Could you check a few things on this model? Use its own coordinates, in mm. A direction names the side the tool comes from. Give positions to 0.01 mm unless a question says otherwise; leave off trailing zeros. Loops run counter-clockwise (first coordinate to the right, second up) from the corner with the lowest first, then second, coordinate; pieces in that order, holes last. Notation, with made-up numbers: (22, 57.5) -> (73, 57.5) arc R27 ccw to (73, 95.5) -> close; hole circle Ø2 at (58, 33.5). An arc over 180 degrees is marked (long way). Write item = value, one per line. Start each with the question number.
1) I want a section at D-D (z = -11). List the corners of the cut face in (x, y) for me (3 decimals).
2) I'm going to push flat-ended pins straight in: pin 1 Ø3 at (x, z) = (15.875, -6.35) entering from -Y; pin 2 Ø5 at (x, y) = (35.5, 31.5) entering from -Z. Where does each tip first touch, or does it pass through?
3) I want a section at B-B (y = 24.13). List the corners of the cut face in (x, z) for me (3 decimals).
4) I want a section at C-C (x = 6.35). List the corners of the cut face in (y, z) for me (3 decimals), and give its area (3 significant figures).
5) On a 3-axis mill with a long thin cutter (end or side, diameter ignored), from which of +Z, -Z, +X, -X, +Y, -Y can I reach the whole of each face in a straight line? I mean faces 1 (the face through (6, 6, -10.16)), 2 (the face through (38.1, 25, -19)), 3 (the face through (6.6, 45.07, -12.88)), 4 (the face through (14.015, 8.766, -5.937)). Say none if no direction works.
6) I need wall thicknesses on probe 1 along Y at (x, z) = (6.35, -16.75) (3 decimals); probe 2 along X at (y, z) = (47, -18.5); probe 3 along X at (y, z) = (6.5, -15). Which ranges of each line are inside material? Lowest first, please. Write a range as from..to.
7) If we mould it in two halves opening along X, with no side actions, what happens to faces 5 (the face through (35, 25, -12.7)), 6 (the face through (25.49, 29.32, -17.54)), 7 (the face through (50.8, 25, -13))? For each: +X half, -X half, draft (parallel to the pull), parting line (faces both ways), or undercut.
8) I want a section at A-A (z = -16.5). Count the separate pieces of the cut face and the enclosed holes in it, and give its area (3 significant figures).
from build123d import *

# Parameters (mm, degrees)
BOSS_EXTRUDE1_DEPTH = 50.8
SKETCH2_R           = 1.75
CUT_EXTRUDE1_DEPTH  = 15.24
CUT_EXTRUDE2_REACH  = 78.2
SKETCH4_R           = 1.905
SKETCH5_R           = 1.905
CUT_EXTRUDE3_DEPTH  = 25.4
SKETCH6_R           = 1.905
CUT_EXTRUDE4_DEPTH  = 17.78


with BuildPart() as part:
    # Sketch1 → Boss-Extrude1 (new body)
    with BuildSketch(Plane(origin=(0, 0, 0), x_dir=(1, 0, 0), z_dir=(0, 1, 0))):
        Polygon((0, 0), (0, 25.4), (12.7, 25.4), (12.7, 12.7), (19.05, 12.7), (19.05, 25.4), (31.75, 25.4), (31.75, 12.7), (38.1, 12.7), (38.1, 25.4), (50.8, 25.4), (50.8, 0), align=None)
    extrude(amount=BOSS_EXTRUDE1_DEPTH)

    # Sketch2 → Cut-Extrude1 (cut)
    with BuildSketch(Plane(origin=(0, 0, -25.4), x_dir=(-1, 0, 0), z_dir=(0, 0, -1))):
        with Locations((-44.45, 6.35)):
            Circle(SKETCH2_R)
        with Locations((-6.35, 6.35)):
            Circle(SKETCH2_R)
    extrude(amount=-CUT_EXTRUDE1_DEPTH, mode=Mode.SUBTRACT)

    # Cut-Extrude2: up to this face of the body (flat: up to its plane)
    cut_extrude2_end = Plane(part.part.faces().sort_by_distance((0, 25.4, -12.7))[0])
    # Sketch4 → Cut-Extrude2 (cut, up to the picked face)
    with BuildSketch(Plane(origin=(50.8, 0, 0), x_dir=(0, 0, -1), z_dir=(1, 0, 0)), mode=Mode.PRIVATE) as cut_extrude2_sk1:
        with Locations((19.05, 30.48)):
            Circle(SKETCH4_R)
    cut_extrude2_tool1 = split(extrude(cut_extrude2_sk1.sketch, amount=-CUT_EXTRUDE2_REACH, mode=Mode.PRIVATE), bisect_by=cut_extrude2_end, keep=Keep.BOTH, mode=Mode.PRIVATE)
    add(cut_extrude2_tool1.solids().sort_by(Axis((50.8, 30.48, -19.05), (-1, 0, 0)))[0], mode=Mode.SUBTRACT)

    # Sketch5 → Cut-Extrude3 (cut)
    with BuildSketch(Plane(origin=(0, 0, -25.4), x_dir=(-1, 0, 0), z_dir=(0, 0, -1))):
        with Locations((-44.45, 24.13)):
            Circle(SKETCH5_R)
        with Locations((-44.45, 43.18)):
            Circle(SKETCH5_R)
        with Locations((-6.35, 24.13)):
            Circle(SKETCH5_R)
        with Locations((-6.35, 43.18)):
            Circle(SKETCH5_R)
    extrude(amount=-CUT_EXTRUDE3_DEPTH, mode=Mode.SUBTRACT)

    # Sketch6 → Cut-Extrude4 (cut)
    with BuildSketch(Plane.XZ):
        with Locations(Location((34.925, -6.35, 0), (0, 0, 270))):
            Circle(SKETCH6_R)
        with Locations(Location((15.875, -6.35, 0), (0, 0, 270))):
            Circle(SKETCH6_R)
        with Locations(Location((25.4, -19.05, 0), (0, 0, 270))):
            Circle(SKETCH6_R)
    extrude(amount=-CUT_EXTRUDE4_DEPTH, mode=Mode.SUBTRACT)


solid = part.part
Answer list:
q1.outline = (0, 0) -> (50.8, 0) -> (50.8, 50.8) -> (0, 50.8) -> close; hole circle Ø3.81 at (6.35, 24.13); hole circle Ø3.81 at (6.35, 43.18); hole circle Ø3.5 at (6.35, 6.35); hole circle Ø3.81 at (44.45, 24.13); hole circle Ø3.81 at (44.45, 43.18); hole circle Ø3.5 at (44.45, 6.35)
q2.pin_1 = 17.78
q2.pin_2 = -12.7
q3.outline = (0, -25.4) -> (4.445, -25.4) -> (4.445, 0) -> (0, 0) -> close; (8.255, -25.4) -> (12.7, -25.4) -> (12.7, -12.7) -> (19.05, -12.7) -> (19.05, -25.4) -> (31.75, -25.4) -> (31.75, -12.7) -> (38.1, -12.7) -> (38.1, -25.4) -> (42.545, -25.4) -> (42.545, 0) -> (8.255, 0) -> close; (46.355, -25.4) -> (50.8, -25.4) -> (50.8, 0) -> (46.355, 0) -> close
q4.outline = (0, -25.4) -> (4.6, -25.4) -> (4.6, -10.16) -> (8.1, -10.16) -> (8.1, -25.4) -> (22.225, -25.4) -> (22.225, 0) -> (0, 0) -> close; (26.035, -25.4) -> (41.275, -25.4) -> (41.275, 0) -> (26.035, 0) -> close; (45.085, -25.4) -> (50.8, -25.4) -> (50.8, 0) -> (45.085, 0) -> close; hole circle Ø3.81 at (30.48, -19.05)
q4.area = 1,030 mm^2
q5.face_1 = -Z
q5.face_2 = -Z, +Y, -Y
q5.face_3 = +Z, -Z
q5.face_4 = -Y
q6.probe_1 = 0..4.6, 8.1..22.225, 26.035..41.275, 45.085..50.8
q6.probe_2 = 0..12.7, 19.05..31.75, 38.1..50.8
q6.probe_3 = 0..4.61, 8.09..12.7, 19.05..31.75, 38.1..42.71, 46.19..50.8
q7.face_5 = undercut
q7.face_6 = draft
q7.face_7 = +X half
q8.separate_pieces = 3
q8.enclosed_holes = 6
q8.area = 1,870 mm^2
